Read the model definition and answer for the solid it produces. Units are mm, in the model's axes. Face numbers are marked on the shaded views. A direction names the side the tool comes from. Coordinates: 2 decimals unless noted, no trailing zeros. Loops run counter-clockwise (first coordinate to the right, second up) from the corner with the lowest first, then second, coordinate; pieces in that order, holes last. Notation, with made-up numbers: M -7.75,63 L 45.25,63 A17 ccw 45.25,70 Z; hole C 4.25,-30.5 d4. An arc over 180 degrees is marked long. One line per item, written item: value. Start each with the question number.
```python
from build123d import *

# Parameters (mm, degrees)
F1_DEPTH = 15
F0_R     = 10
F2_DEPTH = 3
F4_DEPTH = 11
F5_DEPTH = 3


with BuildPart() as f1:
    # F0 (on Top) → F1 (new body)
    with BuildSketch(Plane.XY):
        with BuildLine():
            add(Edge.make_bspline(
                [(25, 0), (25.0087002696, -5.8990169969), (22.1552822861, -16.7434149041), (11.7382328833, -28.4109430259), (2.8895078726, -33.2599749563), (-2.8164344422, -34.2581364978), (-6.2585137784, -34.5978120347)],
                knots=[0, 0, 0, 0, 0.2908567046, 0.5661013385, 0.7856454444, 1, 1, 1, 1], degree=3))
            ThreePointArc((25, 0), (-8.821991792, 23.3917177826), (-18.7737968657, -16.5089233823))
            Line((-18.7737968657, -16.5089233823), (-27.0137283951, -16.5089233823))
            Line((-27.0137283951, -16.5089233823), (-27.0137283951, -20.5689330128))
            Line((-27.0137283951, -20.5689330128), (-23.3377733697, -20.5689330128))
            Line((-23.3377733697, -20.5689330128), (-14.2098203618, -20.5689330128))
            Line((-14.2098203618, -20.5689330128), (-6.2585137784, -20.5689330128))
            ThreePointArc((-6.2585137784, -20.5689330128), (-12.8002334698, 17.2743747533), (21.5, 0))
            ThreePointArc((21.5, 0), (13.189427122, -20.3534456592), (-6.2585137784, -30.6055657566))
            Line((-6.2585137784, -30.6055657566), (-23.3377733697, -30.6055657566))
            Line((-23.3377733697, -30.6055657566), (-27.0137283951, -30.6055657566))
            Line((-27.0137283951, -30.6055657566), (-27.0137283951, -34.5978120347))
            Line((-27.0137283951, -34.5978120347), (-6.2585137784, -34.5978120347))
        make_face()
    extrude(amount=F1_DEPTH)

    # F0 (on Top) → F2 (join)
    with BuildSketch(Plane.XY):
        with BuildLine():
            Line((-23.3377733697, -20.5689330128), (-27.0137283951, -20.5689330128))
            Line((-27.0137283951, -20.5689330128), (-27.0137283951, -21.3873516768))
            Line((-27.0137283951, -21.3873516768), (-27.0137283951, -30.6055657566))
            Line((-27.0137283951, -30.6055657566), (-23.3377733697, -30.6055657566))
            Line((-23.3377733697, -30.6055657566), (-6.2585137784, -30.6055657566))
            ThreePointArc((-6.2585137784, -30.6055657566), (13.189427122, -20.3534456592), (21.5, 0))
            ThreePointArc((21.5, 0), (-12.8002334698, 17.2743747533), (-6.2585137784, -20.5689330128))
            Line((-6.2585137784, -20.5689330128), (-14.2098203618, -20.5689330128))
            Line((-14.2098203618, -20.5689330128), (-23.3377733697, -20.5689330128))
        make_face()
        with Locations((0.5567180342, 0)):
            Circle(F0_R, mode=Mode.SUBTRACT)
    extrude(amount=F2_DEPTH)

    # F3 (on face) → F4 (join)
    with BuildSketch(Plane(origin=(0, -30.6055657566, 0), x_dir=(-1, 0, 0), z_dir=(0, 1, 0))):
        with BuildLine():
            add(Edge.make_bspline(
                [(18.3209385723, 3), (19.5423853219, 3.4077423094), (23.2709452392, 5.8971211647), (25.1604775917, 9.372303958), (26.423119613, 12.9164144641), (27.0137283951, 15)],
                knots=[0, 0, 0, 0, 0.3426311752, 0.6413082257, 1, 1, 1, 1], degree=3))
            Line((18.3209385723, 3), (27.0137283951, 3))
            Line((27.0137283951, 3), (27.0137283951, 15))
        make_face()
    extrude(amount=F4_DEPTH)

    # F5 (add): a face of the model
    f5_faces = [f1.faces().sort_by_distance(p)[0] for p in [
        (-27.0137283951, -25.5533677085, 7.5),
    ]]
    extrude(f5_faces, amount=F5_DEPTH)


solid = f1.part
```
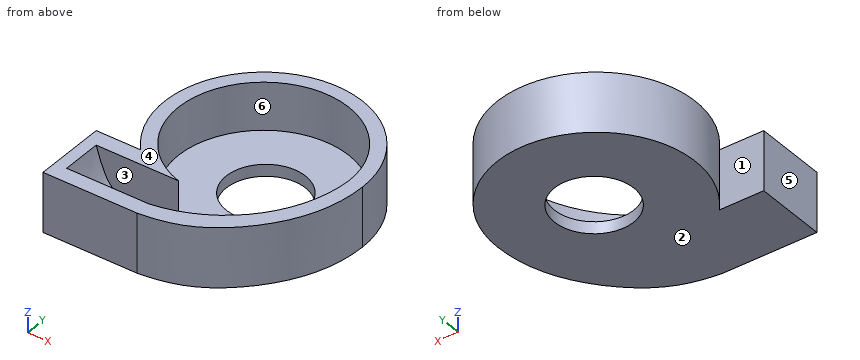
1) Section A-A (y = 5) is taken. Determine the outline of the cut face in (x, z), then the cut area to 3 significant figures.
2) A tool of negligible diameter and unlimited length cuts with its end or side. For the marked faces 1, 2 and 3, from which of +Z, -Z, +X, -X, +Y, -Y can it reach the whole face along a straight path? Write none if from no direction.
3) Section C-C (y = 17) is taken. Determine the outline of the cut face in (x, z), then the cut area to 3 significant figures.
4) For a pull along X with two mould halves and no side action, classify the marked faces 4, 5 and 6 as released by +X, released by -X, zero draft, split by the parting line, or undercut.
5) Consider line 1 along X through (y, z) = (0, 7); line 2 along Z through (x, y) = (-10, 1.5); line 3 along Y through (x, z) = (0, 6.5). Determine where each line is inside the solid, lowest interval first.
6) Flat-ended cylindrical pins translate along their axes: pin 1 (6 mm diameter, centred on x = 17, z = 11.5, fed in from +Y); pin 2 (1 mm diameter, centred on x = -6, y = -24, fed in from -Z); pin 3 (4 mm diameter, centred on x = -23.5, z = 4, fed in from +Y); pin 4 (1.5 mm diameter, centred on y = 6.5, z = 10, fed in from +X). Find the tip coordinate at first contact, or state that the pin passes through.
7) Section B-B (x = -8) is taken. Determine the outline of the cut face in (y, z), then the cut area to 3 significant figures.
Results found:
1. outline: M -24.49,0 L -8.1,0 L -8.1,3 L -20.91,3 L -20.91,15 L -24.49,15 Z; M 9.22,0 L 24.49,0 L 24.49,15 L 20.91,15 L 20.91,3 L 9.22,3 Z
1. area: 181 mm²
2. face 1: +Z, -Z, -X
2. face 2: -Z, +X, -X, +Y, -Y
2. face 3: +Z
3. outline: M -18.33,0 L 18.33,0 L 18.33,15 L 13.16,15 L 13.16,3 L -13.16,3 L -13.16,15 L -18.33,15 Z
3. area: 234 mm²
4. face 4: zero draft
4. face 5: released by -X
4. face 6: undercut
5. line 1: x = -25 to -21.5, 21.5 to 25
5. line 2: z = 0 to 3
5. line 3: y = -33.61 to -29.1, 21.5 to 25
6. pin 1: stops at y = 20.71
6. pin 2: stops at z = 0
6. pin 3: stops at y = 12.76
6. pin 4: stops at x = 24.33
7. outline: M -34.6,0 L -5.18,0 L -5.18,3 L -19.96,3 L -19.96,15 L -20.57,15 L -20.57,3 L -30.61,3 L -30.61,15 L -34.6,15 Z; M 5.18,0 L 23.69,0 L 23.69,15 L 19.96,15 L 19.96,3 L 5.18,3 Z
7. area: 244 mm²
